CAD build for the part. Positions are in the model's coordinates, mm. Give positions to 0.01 mm unless a question says otherwise; leave off trailing zeros. Loops run counter-clockwise (first coordinate to the right, second up) from the corner with the lowest first, then second, coordinate; pieces in that order, holes last. Notation, with made-up numbers: (64, -37) -> (81, -37) arc R11 ccw to (81, -26) -> close; hole circle Ø3 at (-29, -25.75). An arc over 180 degrees is marked (long way). Write each question's results on one line, items separated by ' | '. Start each with the question number.
```python
from build123d import *

# Parameters (mm, degrees)
SKETCH2_W           = 653.034
SKETCH2_H           = 358.648
BOSS_EXTRUDE1_DEPTH = 57.15
SKETCH3_W           = 526.034
SKETCH3_H           = 31.75
CUT_EXTRUDE1_DEPTH  = 25.4
SKETCH4_R           = 9.525
BOSS_EXTRUDE2_DEPTH = 25.4
FILLET1_R           = 25.4


with BuildPart() as part:
    # Sketch2 → Boss-Extrude1 (new body)
    with BuildSketch(Plane(origin=(0, 0, 0), x_dir=(1, 0, 0), z_dir=(0, 1, 0))):
        Rectangle(SKETCH2_W, SKETCH2_H)
    extrude(amount=BOSS_EXTRUDE1_DEPTH)

    # Sketch3 → Cut-Extrude1 (cut)
    with BuildSketch(Plane(origin=(0, 0, -179.324), x_dir=(-1, 0, 0), z_dir=(0, 0, -1))):
        with Locations((0, 15.875)):
            Rectangle(SKETCH3_W, SKETCH3_H)
    extrude(amount=-CUT_EXTRUDE1_DEPTH, mode=Mode.SUBTRACT)

    # Sketch4 → Boss-Extrude2 (add)
    with BuildSketch(Plane.ZY.offset(-263.017)):
        with Locations(Location((-165.585268519, 17.143786042, 0), (0, 0, 180))):
            Circle(SKETCH4_R)
    boss_extrude2 = extrude(amount=BOSS_EXTRUDE2_DEPTH)

    # Mirror1: Boss-Extrude2 across plane
    add(boss_extrude2.mirror(Plane.ZY))

    # Fillet1
    fillet1_edges = [part.edges().sort_by_distance(p)[0] for p in [
        (-294.767, 0, -179.324),
        (294.767, 0, -179.324),
    ]]
    fillet(fillet1_edges, radius=FILLET1_R)


solid = part.part
```
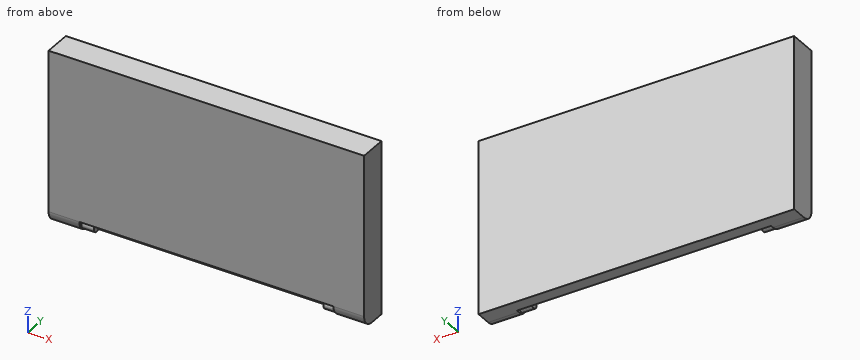
Q1. Saw through at A-A, the plane x = -249. List the corners of the cut face in (y, z) (3 decimals).
Q2. Wall check: L1, parallel to Z at x = 191, y = 3.5; L2, parallel to X at y = 18, z = -158.5; L3, parallel to Y at x = 78, z = -158. Give the ranges that are in metal, low to high.
Q3. Saw through at B-B, the plane x = -81. List the corners of the cut face in (y, z), then the cut area to 3 significant figures.
Answer block:
1) outline: (0, -153.924) -> (31.75, -153.924) -> (31.75, -179.324) -> (57.15, -179.324) -> (57.15, 179.324) -> (0, 179.324) -> close; circle Ø19.05 at (17.144, -165.585)
2) L1: z = -153.92 to 179.32 | L2: x = -326.52 to -237.62, 237.62 to 326.52 | L3: y = 31.75 to 57.15
3) outline: (0, -153.92) -> (31.75, -153.92) -> (31.75, -179.32) -> (57.15, -179.32) -> (57.15, 179.32) -> (0, 179.32) -> close | area: 19,700 mm2
